Part model, mm, in its own coordinate system. Face numbers are marked on the shaded views. A direction names the side the tool comes from. Coordinates: 2 decimals unless noted, no trailing zeros. Loops run counter-clockwise (first coordinate to the right, second up) from the corner with the lowest first, then second, coordinate; pieces in that order, holes last. Notation, with made-up numbers: M -23,85 L 9,85 A10 ccw 9,94 Z; hole C 86,57 d9. An arc over 180 degrees is marked long. Use a Markdown table: item, result. Add a question column.
1) Band-saw the part on B-B (y = 4). List the corners of the cut face in (x, z).
2) Pin check, flat tips, straight feed: pin 1 Ø4.5 at (y, z) = (-6.5, 6.5) entering from -X; pin 2 Ø0.9 at (x, z) = (10, 4) entering from +Y; pin 3 Ø2 at (x, y) = (13, 4) entering from -Z; pin 4 Ø10 at (x, y) = (-7, 8) entering from +Z. Stop position of each tip, or through.
3) Wall check: probe 1 along Y at (x, z) = (19, 13.55) (3 decimals); probe 2 along Y at (x, z) = (8.5, 7.25); probe 3 along Z at (x, y) = (-22, 7). Give the ranges that are in metal, low to high. Write a range as from..to.
4) Band-saw the part on C-C (z = 7.5). List the corners of the cut face in (x, y).
5) Band-saw the part on A-A (x = 19). List the corners of the cut face in (y, z) (3 decimals), plus the area to 3 significant figures.
6) Pull direction Z, two halves, no side cores. Call the marked faces 4, 5 and 6: released by +Z, released by -Z, zero draft, split by the parting line, or undercut.
7) Band-saw the part on D-D (x = -13). List the corners of the cut face in (y, z) (3 decimals), plus the area to 4 significant figures.
8) Tool access for the marked faces 1, 2 and 3: list every direction of +Z, -Z, +X, -X, +Y, -Y with a clear straight run to the whole face (end or side of a thin tool).
from build123d import *

# Parameters (mm, degrees)
F0_W     = 13.375
F0_H     = 2
F1_DEPTH = 25
F2_R     = 1.75
F3_DEPTH = 2
F5_DEPTH = 30
F6_W     = 5
F6_H     = 8
F7_DEPTH = 50.001
F8_R     = 1.6
F9_DEPTH = 2.5
F10_R    = 7.5
F11_R    = 3
F12_R    = 2
F13_SIZE = 0.4


with BuildPart() as f1:
    # F0 (on Right) → F1 (new body, symmetric)
    with BuildSketch(Plane.YZ):
        with Locations((6.6875, 1)):
            Rectangle(F0_W, F0_H)
    extrude(amount=F1_DEPTH, both=True)

    # F2 (on face) → F3 (cut, through all)
    with BuildSketch(Plane.XY.offset(2)):
        with Locations((-13, 4)):
            Circle(F2_R)
        with Locations((13, 4)):
            Circle(F2_R)
    extrude(amount=-F3_DEPTH, mode=Mode.SUBTRACT)

    # F4 (on face) → F5 (join)
    with BuildSketch(Plane.YZ.offset(25)):
        Polygon((-10, 0), (0, 0), (0, 15.3), (-25, 15.3), (-25, 12.8), (-10, 12.8), align=None)
    extrude(amount=-F5_DEPTH)

    # F6 (on face) → F7 (cut, through all)
    with BuildSketch(Plane.YZ.offset(25)):
        with Locations((-2.5, 9)):
            Rectangle(F6_W, F6_H)
    extrude(amount=-F7_DEPTH, mode=Mode.SUBTRACT)

    # F8 (on face) → F9 (cut, through all)
    with BuildSketch(Plane(origin=(0, 0, 12.8), x_dir=(1, 0, 0), z_dir=(0, 0, -1))):
        with Locations((1, 19.235)):
            Circle(F8_R)
        with Locations((19, 19.235)):
            Circle(F8_R)
    extrude(amount=-F9_DEPTH, mode=Mode.SUBTRACT)

    # F10
    f10_edges = [f1.edges().sort_by_distance(p)[0] for p in [
        (-5, -25, 14.05),
    ]]
    fillet(f10_edges, radius=F10_R)

    # F11
    f11_edges = [f1.edges().sort_by_distance(p)[0] for p in [
        (10, -10, 12.8),
    ]]
    fillet(f11_edges, radius=F11_R)

    # F12
    f12_edges = [f1.edges().sort_by_distance(p)[0] for p in [
        (-5, 0, 1),
    ]]
    fillet(f12_edges, radius=F12_R)

    # F13
    f13_edges = [f1.edges().sort_by_distance(p)[0] for p in [
        (25, -10, 4.9),
        (25, -10.87868, 11.92132),
        (25, 1.6875, 0),
        (25, -19, 12.8),
        (25, 13.375, 1),
        (25, -25, 14.05),
        (25, 6.6875, 2),
        (25, -12.5, 15.3),
        (25, 0, 3.5),
        (25, 0, 14.15),
        (25, -2.5, 5),
        (25, -2.5, 13),
        (25, -5, 9),
    ]]
    chamfer(f13_edges, length=F13_SIZE)


solid = f1.part
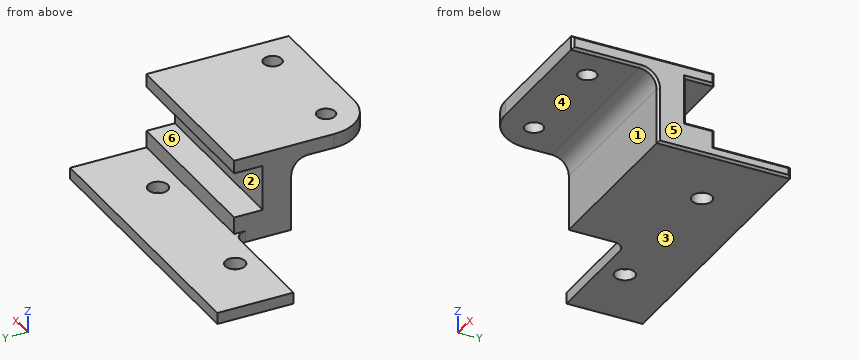
Entries:
| question | item | result |
|---|---|---|
| 1 | outline | M -25,0 L -14.75,0 L -14.75,2 L -25,2 Z; M -11.25,0 L 11.25,0 L 11.25,2 L -11.25,2 Z; M 14.75,0 L 24.6,0 L 25,0.4 L 25,1.6 L 24.6,2 L 14.75,2 Z |
| 2 | pin 1 | x = -5 |
| 2 | pin 2 | y = 0 |
| 2 | pin 3 | through |
| 2 | pin 4 | z = 2 |
| 3 | probe 1 | -25..-20.835, -17.635..0 |
| 3 | probe 2 | -10..-5 |
| 3 | probe 3 | 0..2 |
| 4 | outline | M -5,-10 L 24.6,-10 L 25,-9.6 L 25,-5.4 L 24.6,-5 L -5,-5 Z |
| 5 | outline | M -25,12.8 L -20.835,12.8 L -20.835,15.3 L -25,15.3 Z; M -17.635,12.8 L -13,12.8 A3 cw -10,9.8 L -10,0 L 13.375,0 L 13.375,2 L 0,2 L 0,5 L -5,5 L -5,13 L 0,13 L 0,15.3 L -17.635,15.3 Z |
| 5 | area | 171 mm2 |
| 6 | face 4 | released by -Z |
| 6 | face 5 | zero draft |
| 6 | face 6 | undercut |
| 7 | outline | M 0,0 L 2.25,0 L 2.25,2 L 0,2 Z; M 5.75,0 L 13.375,0 L 13.375,2 L 5.75,2 Z |
| 7 | area | 19.75 mm2 |
| 8 | face 1 | -Z, +X, -X, -Y |
| 8 | face 2 | +X, -X, +Y |
| 8 | face 3 | -Z, +X, -X, +Y, -Y |
